Solid Edge part; units mm, degrees
sketch "Sketch1" plane through (0, 0, 0) normal (0, -1, 0) x (1, 0, 0)
  line L0 (4, 0) -> (1.8, 0)
  line L1 (1.8, 0) -> (1.8, -1.4)
  line L2 (1.8, -1.4) -> (2, -1.4)
  line L3 (2, -1.4) -> (2, -10)
  line L4 (2, -10) -> (0, -10)
  arc A0 (0, 3.1) -> (4, 2.0282) centre (0, -4.9) cw
  line L5 (4, 0) -> (4, 2.0282)
  dimension "D1" = 1.8
  dimension "D2" = 1.8
revolve "RevolvedProtrusion1" add sketch "Sketch1" angle 360 about axis through (0, 0, -6) along (0, 0, 1)
cosmetic_thread "Thread1"
chamfer "Chamfer_1" distance 0.4 angle 45 1 edges at (-2, 0, -10)
fillet "Round1" radius 0.2 2 edges at (-1.8, 0, -1.4) (-1.8, 0, 0)
fillet "Round_3" radius 1 1 edges at (-4, 0, 2.0282)
sketch "Sketch2" plane through (0, 0, 3.1) normal (0, 0, 1) x (1, 0, 0)
  line L0 (-0.5, 0.5) -> (-0.5, 2.3)
  line L1 (-0.5, 2.3) -> (0.5, 2.3)
  line L2 (0.5, 2.3) -> (0.5, 0.5)
  line L3 (0.5, 0.5) -> (2.3, 0.5)
  line L4 (2.3, 0.5) -> (2.3, -0.5)
  line L5 (2.3, -0.5) -> (0.5, -0.5)
  line L6 (0.5, -0.5) -> (0.5, -2.3)
  line L7 (0.5, -2.3) -> (-0.5, -2.3)
  line L8 (-0.5, -2.3) -> (-0.5, -0.5)
  line L9 (-0.5, -0.5) -> (-2.3, -0.5)
  line L10 (-2.3, -0.5) -> (-2.3, 0.5)
  line L11 (-2.3, 0.5) -> (-0.5, 0.5)
  dimension "D1" = 0.5
extrude "ExtrudedCutout_2" cut sketch "Sketch2" against normal blind 2.3
properties part number "STD-DIN7985-M4x10" material "Galvanized steel"
The listing builds one solid part. Answer for the finished solid, in the listing's coordinates (mm). A direction names the side the tool comes from. Give positions to 0.01 mm unless a question says otherwise; leave off trailing zeros. Order: outer loops, then holes, each group sorted by start corner. A loop starts at its lowest first (then second) coordinate and runs counter-clockwise, first axis right, second up. Notation, with made-up numbers: (10, 38.5) - (60, 38.5) arc R22 cw to (60, 44.5) - close; hole circle Ø9 at (50, 44). An arc over 180 degrees is marked (long way). Use one line per item in the form item = value. Start each with the question number.
(1) A cutting plane is placed at A-A, the plane z = 0.25. Write down the section's boundary in (x, y), then the cut area to 3 significant figures.
(2) A cutting plane is placed at B-B, the plane z = -4.75. Write down the section's boundary in (x, y).
(3) The mould has two halves that part along Y. Classify faces 3 (the flat face through (2.3, 0, 2)), 4 (the cylindrical face through (0, 2, -6)), 5 (the flat face through (-2, -1, 0)): released by +Y, released by -Y, zero draft, split by the parting line, or undercut.
(4) Consider line 1 (X direction, y = 1.5, z = 2); line 2 (X direction, y = -0.75, z = 1.75); line 3 (Y direction, x = 0, z = -4). Determine where each line is inside the solid, lowest interval first. Write a range as from..to.
(5) For faces 1 (the cylindrical face through (-0.867, -3.905, 0.722)), 2 (the flat face through (0, 2.3, 2)), determine the directions among +Z, -Z, +X, -X, +Y, -Y from which every point of the face is accessible in a straight line to the end or side of a thin tool.
(6) Flat-ended cylindrical pins translate along their axes: pin 1 Ø1.5 at (y, z) = (1.5, -5) entering from -X; pin 2 Ø1.4 at (y, z) = (1, 2) entering from +X; pin 3 Ø1.4 at (x, z) = (1.5, 2) entering from +Y. Find the tip coordinate at first contact, or state that the pin passes through.
Ans:
q1.outline = circle Ø8 at (0, 0)
q1.area = 50.3 mm^2
q2.outline = circle Ø4 at (0, 0)
q3.face_3 = undercut
q3.face_4 = split by the parting line
q3.face_5 = zero draft
q4.line_1 = -3.51..-0.5, 0.5..3.51
q4.line_2 = -3.87..-0.5, 0.5..3.87
q4.line_3 = -2..2
q5.face_1 = +Z, -Z
q5.face_2 = +Z
q6.pin_1 = -1.85
q6.pin_2 = 3.97
q6.pin_3 = 3.88
